Geometry check sheet. Reference: the model listing, model coordinates, mm. Face numbers are marked on the shaded views. A direction names the side the tool comes from. Give positions to 0.01 mm unless a question says otherwise; leave off trailing zeros. Loops run counter-clockwise (first coordinate to the right, second up) from the corner with the lowest first, then second, coordinate; pieces in that order, holes last.
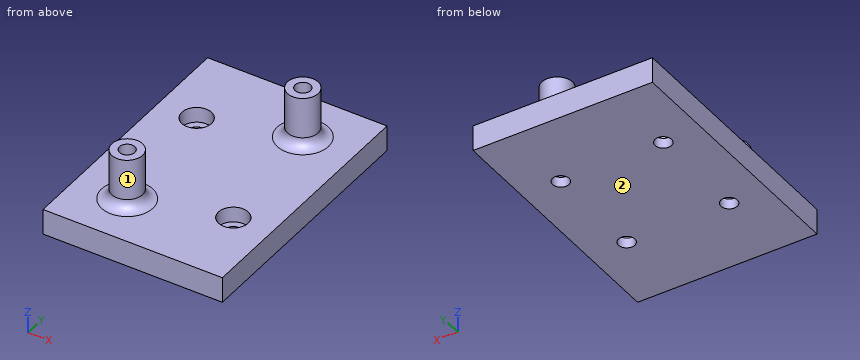
```python
from build123d import *

# Parameters (mm, degrees)
SKETCH_W        = 35
SKETCH_H        = 50
PAD_DEPTH       = 5
SKETCH004_R     = 2.9
POCKET_DEPTH    = 3
SKETCH005_R     = 1.6
POCKET001_DEPTH = 5
SKETCH006_R     = 3
PAD001_DEPTH    = 10
SKETCH007_R     = 1.5
POCKET002_DEPTH = 8
FILLET_R        = 2


with BuildPart() as part:
    # Sketch → Pad (new body)
    with BuildSketch(Plane.XY):
        with Locations((17.5, 25)):
            Rectangle(SKETCH_W, SKETCH_H)
    extrude(amount=PAD_DEPTH)

    # Sketch004 → Pocket (cut)
    with BuildSketch(Plane.XY.offset(5)):
        with Locations((7.5, 35)):
            Circle(SKETCH004_R)
        with Locations((27.5, 15)):
            Circle(SKETCH004_R)
    extrude(amount=-POCKET_DEPTH, mode=Mode.SUBTRACT)

    # Sketch005 → Pocket001 (cut)
    with BuildSketch(Plane.XY.offset(2)):
        with Locations((7.5, 15)):
            Circle(SKETCH005_R)
        with Locations((7.5, 35)):
            Circle(SKETCH005_R)
        with Locations((27.5, 15)):
            Circle(SKETCH005_R)
        with Locations((27.5, 35)):
            Circle(SKETCH005_R)
    extrude(amount=-POCKET001_DEPTH, mode=Mode.SUBTRACT)

    # Sketch006 → Pad001 (new body)
    with BuildSketch(Plane.XY.offset(5)):
        with Locations((10, 10)):
            Circle(SKETCH006_R)
        with Locations((25, 40)):
            Circle(SKETCH006_R)
    extrude(amount=PAD001_DEPTH)

    # Sketch007 → Pocket002 (cut)
    with BuildSketch(Plane.XY.offset(15)):
        with Locations((10, 10)):
            Circle(SKETCH007_R)
        with Locations((25, 40)):
            Circle(SKETCH007_R)
    extrude(amount=-POCKET002_DEPTH, mode=Mode.SUBTRACT)

    # Fillet
    fillet_edges = [part.edges().sort_by_distance(p)[0] for p in [
        (22, 40, 5),
        (7, 10, 5),
    ]]
    fillet(fillet_edges, radius=FILLET_R)


solid = part.part
```
1) Depth check by flat-ended pin: P1, Ø5, axis at x = 27.5, y = 15, coming from the +Z side; P2, Ø4.5, axis at x = 8, y = 34.5, coming from the +Z side; P3, Ø0.9, axis at x = 25, y = 39.5, coming from the +Z side. Enter the tip coordinate at first touch or a pass-through.
2) Sectioned sample at B-B on y = 10. Enter the section's corners in (x, z), plus the area to 3 significant figures.
3) Scan lines: line 1 along Y through (x, z) = (27.5, 0.45); line 2 along Y through (x, z) = (10, 11); line 3 along Y through (x, z) = (27.5, 4.05). Record each from-to range of solid material in increasing order.
4) Tool access check on the marked faces 1 and 2. Record the directions out of +Z, -Z, +X, -X, +Y, -Y that give a thin tool (end or side, any length) a straight path to the whole face; none if there is none.
5) Sectioned sample at A-A on z = 1.25. Enter the section's corners in (x, y).
6) Sectioned sample at D-D on y = 30.5. Enter the section's corners in (x, z), plus the area to 3 significant figures.
7) Sectioned sample at C-C on z = 13.75. Enter the section's corners in (x, y).
Determined:
1. P1: stops at z = 2
1. P2: stops at z = 5
1. P3: stops at z = 7
2. outline: (0, 0) - (35, 0) - (35, 5) - (15, 5) arc R2 cw to (13, 7) - (13, 15) - (11.5, 15) - (11.5, 7) - (8.5, 7) - (8.5, 15) - (7, 15) - (7, 7) arc R2 cw to (5, 5) - (0, 5) - close
2. area: 213 mm2
3. line 1: y = 0 to 13.4, 16.6 to 33.4, 36.6 to 50
3. line 2: y = 7 to 8.5, 11.5 to 13
3. line 3: y = 0 to 12.1, 17.9 to 50
4. face 1: +Z
4. face 2: -Z, +X, -X, +Y, -Y
5. outline: (0, 0) - (35, 0) - (35, 50) - (0, 50) - close; hole circle Ø3.2 at (7.5, 15); hole circle Ø3.2 at (7.5, 35); hole circle Ø3.2 at (27.5, 15); hole circle Ø3.2 at (27.5, 35)
6. outline: (0, 0) - (35, 0) - (35, 5) - (0, 5) - close
6. area: 175 mm2
7. outline: circle Ø6 at (10, 10); circle Ø6 at (25, 40); hole circle Ø3 at (10, 10); hole circle Ø3 at (25, 40)
